Part model, mm, in its own coordinate system. A direction names the side the tool comes from. Give positions to 0.01 mm unless a question says otherwise; leave off trailing zeros. Order: outer loops, then holes, each group sorted by start corner. A loop starts at its lowest first (then second) coordinate and runs counter-clockwise, first axis right, second up. Notation, with made-up numbers: M -13,42.5 L 43,42.5 A21 ccw 43,60.5 Z; hole C -23,29.25 d9. An arc over 180 degrees is marked long. One line per question, with ' | ' between items.
```python
from build123d import *

# Parameters (mm, degrees)
SKETCH1_W           = 9
SKETCH1_H           = 40
BOSS_EXTRUDE1_DEPTH = 2.5
SKETCH2_R           = 2.5
BOSS_EXTRUDE2_DEPTH = 40
CUT_EXTRUDE1_START  = -4.75
SKETCH3_R           = 2.875
CUT_EXTRUDE1_DEPTH  = 10.5
BOSS_EXTRUDE3_REACH = 28.806
SKETCH4_R           = 1
SKETCH5_R           = 1
CUT_EXTRUDE2_DEPTH  = 42.076148797
CHAMFER1_SIZE       = 1.5
CHAMFER2_SIZE       = 1.5
SKETCH6_W           = 6.5
SKETCH6_H           = 0.2
CUT_EXTRUDE3_DEPTH  = 42.303752856
SKETCH7_R           = 1.25
CUT_EXTRUDE4_DEPTH  = 1
CHAMFER3_SIZE       = 1


with BuildPart() as part:
    # Sketch1 → Boss-Extrude1 (new body)
    with BuildSketch(Plane(origin=(0, 0, 0), x_dir=(1, 0, 0), z_dir=(0, 1, 0))):
        with Locations((-4.5, 20)):
            Rectangle(SKETCH1_W, SKETCH1_H)
    extrude(amount=BOSS_EXTRUDE1_DEPTH)

    # Sketch2 → Boss-Extrude2 (add)
    with BuildSketch(Plane.XY):
        with Locations((0, 2.5)):
            Circle(SKETCH2_R)
    extrude(amount=-BOSS_EXTRUDE2_DEPTH)

    # Sketch3 → Cut-Extrude1 (cut)
    with BuildSketch(Plane.XY.offset(CUT_EXTRUDE1_START)):
        with Locations((0, 2.5)):
            Circle(SKETCH3_R)
    cut_extrude1 = extrude(amount=-CUT_EXTRUDE1_DEPTH, mode=Mode.SUBTRACT)

    # Mirror1: Cut-Extrude1 across plane
    add(cut_extrude1.mirror(Plane.XY.offset(-20)), mode=Mode.SUBTRACT)

    # Sketch4 → Boss-Extrude3 (add, up to next)
    with BuildSketch(Plane.XY.offset(-15.25), mode=Mode.PRIVATE) as boss_extrude3_sk1:
        with Locations((0, 2.5)):
            Circle(SKETCH4_R)
    boss_extrude3_tool1 = extrude(boss_extrude3_sk1.sketch, amount=BOSS_EXTRUDE3_REACH, mode=Mode.PRIVATE) - part.part
    boss_extrude3 = boss_extrude3_tool1.solids().sort_by_distance((0, 2.5, -15.25))[0]
    add(boss_extrude3)

    # Mirror2: Boss-Extrude3 across plane
    add(boss_extrude3.mirror(Plane.XY.offset(-20)))

    # Sketch5 → Cut-Extrude2 (cut, through all)
    with BuildSketch(Plane(origin=(0, 2.5, 0), x_dir=(1, 0, 0), z_dir=(0, 1, 0))):
        with Locations(Location((-6, 5, 0), (0, 0, 270))):
            Circle(SKETCH5_R)
    cut_extrude2 = extrude(amount=-CUT_EXTRUDE2_DEPTH, mode=Mode.SUBTRACT)

    # Mirror3: Cut-Extrude2 across plane
    add(cut_extrude2.mirror(Plane.XY.offset(-20)), mode=Mode.SUBTRACT)

    # Chamfer1
    chamfer1_edges = [part.edges().sort_by_distance(p)[0] for p in [
        (-6, 2.5, -6),
    ]]
    chamfer(chamfer1_edges, length=CHAMFER1_SIZE)

    # Chamfer2
    chamfer2_edges = [part.edges().sort_by_distance(p)[0] for p in [
        (-6, 2.5, -34),
    ]]
    chamfer(chamfer2_edges, length=CHAMFER2_SIZE)

    # Sketch6 → Cut-Extrude3 (cut, through all)
    with BuildSketch(Plane.XY):
        with Locations((-5.75, 2.4)):
            Rectangle(SKETCH6_W, SKETCH6_H)
    extrude(amount=-CUT_EXTRUDE3_DEPTH, mode=Mode.SUBTRACT)

    # Sketch7 → Cut-Extrude4 (cut)
    with BuildSketch(Plane(origin=(0, 2.3, 0), x_dir=(1, 0, 0), z_dir=(0, 1, 0))):
        with Locations(Location((-6, 30, 0), (0, 0, 270))):
            Circle(SKETCH7_R)
        with Locations(Location((-6, 10, 0), (0, 0, 270))):
            Circle(SKETCH7_R)
    extrude(amount=-CUT_EXTRUDE4_DEPTH, mode=Mode.SUBTRACT)

    # Chamfer3
    chamfer3_edges = [part.edges().sort_by_distance(p)[0] for p in [
        (-6, 2.3, -31.25),
        (-6, 2.3, -11.25),
    ]]
    chamfer(chamfer3_edges, length=CHAMFER3_SIZE - 0.0001)  # a hair under: the kernel refuses the full size


solid = part.part
```
1. Slice it at D-D on x = -6. Give the number of separate pieces and of enclosed holes in the cut face, then the cut area to 3 significant figures.
Worked out:
separate pieces: 3 | enclosed holes: 0 | area: 72.4 mm2
2. Tool access for faces 1 (the flat face through (0, 1, -24.75)), 2 (the flat face through (-6, 2.3, -20)), 3 (the cylindrical face through (-2.44, 0.98, -30.07)): list every direction of +Z, -Z, +X, -X, +Y, -Y with a clear straight run to the whole face (end or side of a thin tool).
Worked out:
face 1: none | face 2: +Z, -Z, -X, +Y | face 3: +Y
3. Drop flat-ended pins along their axis: pin 1 (3 mm diameter, centred on x = -6, z = -10, fed in from +Y); pin 2 (0.8 mm diameter, centred on x = -6, z = -10.5, fed in from +Y); pin 3 (5 mm diameter, centred on x = -4.5, z = -13.5, fed in from +Y). Give the stop position or say it passes through.
Worked out:
pin 1: stops at y = 1.55 | pin 2: stops at y = 1.3 | pin 3: stops at y = 2.3
4. Mould opens along Z. For faces 4 (the cylindrical face through (2, 4, -20)), 5 (the cylindrical face through (-0.13, 3.49, -29.93)), 6 (the flat face through (-2, 2, -40)) say: released by +Z, released by -Z, zero draft, split by the parting line, or undercut.
Worked out:
face 4: zero draft | face 5: undercut | face 6: released by -Z
5. Slice it at A-A on x = 1.5. Give the cut face in (y, z).
Worked out:
outline: M 0.5,-40 L 4.5,-40 L 4.5,-35.25 L 0.5,-35.25 Z; M 0.5,-24.75 L 4.5,-24.75 L 4.5,-15.25 L 0.5,-15.25 Z; M 0.5,-4.75 L 4.5,-4.75 L 4.5,0 L 0.5,0 Z
6. Probe L1, parallel to Z at x = -1.5, y = 0.45; L2, parallel to Z at x = -6, y = 1.35; L3, parallel to Z at x = -7.75, y = 2.2. List the from-to ranges inside material, lowest first. Write a range as from..to.
Worked out:
L1: z = -40..-35.25, -24.75..-15.25, -4.75..0 | L2: z = -40..-36.35, -33.65..-31.3, -28.7..-11.3, -8.7..-6.35, -3.65..0 | L3: z = -40..-36.33, -33.67..-31.25, -28.75..-11.25, -8.75..-6.33, -3.67..0
7. Slice it at C-C on y = 0.6. Give the cut face in (x, z), then the cut area to 3 significant figures.
Worked out:
outline: M -9,-40 L 1.62,-40 L 1.62,-35.25 L -2.16,-35.25 L -2.16,-24.75 L 1.62,-24.75 L 1.62,-15.25 L -2.16,-15.25 L -2.16,-4.75 L 1.62,-4.75 L 1.62,0 L -9,0 Z; hole C -6,-35 d2; hole C -6,-5 d2 | area: 339 mm2
